from build123d import *

# Parameters (mm, degrees)
SKETCH1_W                        = 45
SKETCH1_H                        = 115
BASE_FLANGE1_DEPTH               = 2
EDGE_FLANGE1_STRIP_W             = 9.9732
EDGE_FLANGE1_STRIP_H             = 2
EDGE_FLANGE1_STRIP_CUT_DEPTH     = 115
EDGE_FLANGE1_DEPTH               = 115
EDGE_FLANGE2_STRIP_W             = 9.9732
EDGE_FLANGE2_STRIP_H             = 2
EDGE_FLANGE2_STRIP_CUT_DEPTH     = 115
EDGE_FLANGE2_DEPTH               = 115
EDGE_FLANGE3_STRIP_W             = 9.9732
EDGE_FLANGE3_STRIP_H             = 2
EDGE_FLANGE3_STRIP_CUT_DEPTH     = 115
EDGE_FLANGE3_DEPTH               = 115
EDGE_FLANGE4_STRIP_W             = 9.9732
EDGE_FLANGE4_STRIP_H             = 2
EDGE_FLANGE4_STRIP_CUT_DEPTH     = 115
EDGE_FLANGE4_DEPTH               = 115
TAP_DRILL_FOR_M5_TAP1_AT_2_COUNT = 2
TAP_DRILL_FOR_M5_TAP1_AT_2_PITCH = 20
TAP_DRILL_FOR_M5_TAP1_AT_3_COUNT = 2
TAP_DRILL_FOR_M5_TAP1_AT_3_PITCH = 69.48
TAP_DRILL_FOR_M5_TAP1_AT_4_COUNT = 2
TAP_DRILL_FOR_M5_TAP1_AT_4_PITCH = 89.48
TAP_DRILL_FOR_M5_TAP1_AT_5_COUNT = 2
TAP_DRILL_FOR_M5_TAP1_AT_5_PITCH = 114.373614001
TAP_DRILL_FOR_M5_TAP1_AT_6_COUNT = 2
TAP_DRILL_FOR_M5_TAP1_AT_6_PITCH = 99.509414527
TAP_DRILL_FOR_M5_TAP1_AT_7_COUNT = 2
TAP_DRILL_FOR_M5_TAP1_AT_7_PITCH = 73.990899302
TAP_DRILL_FOR_M5_TAP1_AT_8_COUNT = 2
TAP_DRILL_FOR_M5_TAP1_AT_8_PITCH = 71.2366


# Sheet-metal steps are written as plain solids
with BuildPart() as part:
    # Sketch1 → Base-Flange1 (new body)
    with BuildSketch(Plane.XY):
        Rectangle(SKETCH1_W, SKETCH1_H)
    extrude(amount=-BASE_FLANGE1_DEPTH)

    # Edge-Flange1 strip (across the edge) → Edge-Flange1 strip cut (cut)
    with BuildSketch(Plane(origin=(23, 57.5, -2), x_dir=(-1, 0, 0), z_dir=(0, -1, 0))):
        with Locations((-4.25, -1)):
            Rectangle(EDGE_FLANGE1_STRIP_W, EDGE_FLANGE1_STRIP_H)
    extrude(amount=EDGE_FLANGE1_STRIP_CUT_DEPTH, mode=Mode.SUBTRACT)

    # Edge-Flange1 section (across the edge) → Edge-Flange1 (add)
    with BuildSketch(Plane(origin=(23, 57.5, -2), x_dir=(-1, 0, 0), z_dir=(0, -1, 0))):
        with BuildLine():
            Line((-2, 0.7366), (-2, 43))
            Line((-2, 43), (0, 43))
            Line((0, 43), (0, 0.7366))
            ThreePointArc((0, 0.7366), (0.215745145, 0.215745145), (0.7366, 0))
            Line((0.7366, 0), (0.7366, -2))
            ThreePointArc((0.7366, -2), (-1.198468417, -1.198468417), (-2, 0.7366))
        make_face()
    extrude(amount=EDGE_FLANGE1_DEPTH)

    # Edge-Flange2 strip (across the edge) → Edge-Flange2 strip cut (cut)
    with BuildSketch(Plane(origin=(25, -57.5, -45.5), x_dir=(0, 0, 1), z_dir=(0, 1, 0))):
        with Locations((-4.25, -1)):
            Rectangle(EDGE_FLANGE2_STRIP_W, EDGE_FLANGE2_STRIP_H)
    extrude(amount=EDGE_FLANGE2_STRIP_CUT_DEPTH, mode=Mode.SUBTRACT)

    # Edge-Flange2 section (across the edge) → Edge-Flange2 (add)
    with BuildSketch(Plane(origin=(25, -57.5, -45.5), x_dir=(0, 0, 1), z_dir=(0, 1, 0))):
        with BuildLine():
            Line((-2, 0.7366), (-2, 20.5))
            Line((-2, 20.5), (0, 20.5))
            Line((0, 20.5), (0, 0.7366))
            ThreePointArc((0, 0.7366), (0.215745145, 0.215745145), (0.7366, 0))
            Line((0.7366, 0), (0.7366, -2))
            ThreePointArc((0.7366, -2), (-1.198468417, -1.198468417), (-2, 0.7366))
        make_face()
    extrude(amount=EDGE_FLANGE2_DEPTH)

    # Edge-Flange3 strip (across the edge) → Edge-Flange3 strip cut (cut)
    with BuildSketch(Plane(origin=(-23, -57.5, -2), x_dir=(1, 0, 0), z_dir=(0, 1, 0))):
        with Locations((-4.25, -1)):
            Rectangle(EDGE_FLANGE3_STRIP_W, EDGE_FLANGE3_STRIP_H)
    extrude(amount=EDGE_FLANGE3_STRIP_CUT_DEPTH, mode=Mode.SUBTRACT)

    # Edge-Flange3 section (across the edge) → Edge-Flange3 (add)
    with BuildSketch(Plane(origin=(-23, -57.5, -2), x_dir=(1, 0, 0), z_dir=(0, 1, 0))):
        with BuildLine():
            Line((-2, 0.7366), (-2, 43))
            Line((-2, 43), (0, 43))
            Line((0, 43), (0, 0.7366))
            ThreePointArc((0, 0.7366), (0.215745145, 0.215745145), (0.7366, 0))
            Line((0.7366, 0), (0.7366, -2))
            ThreePointArc((0.7366, -2), (-1.198468417, -1.198468417), (-2, 0.7366))
        make_face()
    extrude(amount=EDGE_FLANGE3_DEPTH)

    # Edge-Flange4 strip (across the edge) → Edge-Flange4 strip cut (cut)
    with BuildSketch(Plane(origin=(-25, 57.5, -45.5), x_dir=(0, 0, 1), z_dir=(0, -1, 0))):
        with Locations((-4.25, -1)):
            Rectangle(EDGE_FLANGE4_STRIP_W, EDGE_FLANGE4_STRIP_H)
    extrude(amount=EDGE_FLANGE4_STRIP_CUT_DEPTH, mode=Mode.SUBTRACT)

    # Edge-Flange4 section (across the edge) → Edge-Flange4 (add)
    with BuildSketch(Plane(origin=(-25, 57.5, -45.5), x_dir=(0, 0, 1), z_dir=(0, -1, 0))):
        with BuildLine():
            Line((-2, 0.7366), (-2, 20.5))
            Line((-2, 20.5), (0, 20.5))
            Line((0, 20.5), (0, 0.7366))
            ThreePointArc((0, 0.7366), (0.215745145, 0.215745145), (0.7366, 0))
            Line((0.7366, 0), (0.7366, -2))
            ThreePointArc((0.7366, -2), (-1.198468417, -1.198468417), (-2, 0.7366))
        make_face()
    extrude(amount=EDGE_FLANGE4_DEPTH)

    # Sketch21 → Tap Drill for M5 Tap1 (revolve, cut)
    with BuildSketch(Plane(origin=(-35.6183, 44.74, -45.5), x_dir=(0, -1, 0), z_dir=(1, 0, 0))):
        Polygon((0, 0), (0, 2), (2.1, 2), (2.1, 0.025), (2.125, 0), align=None)
    tap_drill_for_m5_tap1 = revolve(axis=Axis((-35.6183, 44.74, -39.15), (0, 0, -1)), mode=Mode.SUBTRACT)

    # Tap Drill for M5 Tap1 at 2: Tap Drill for M5 Tap1 ×2
    with Locations(*[(0, -i * TAP_DRILL_FOR_M5_TAP1_AT_2_PITCH, 0) for i in range(1, TAP_DRILL_FOR_M5_TAP1_AT_2_COUNT)]):
        add(tap_drill_for_m5_tap1, mode=Mode.SUBTRACT)

    # Tap Drill for M5 Tap1 at 3: Tap Drill for M5 Tap1 ×2
    with Locations(*[(0, -i * TAP_DRILL_FOR_M5_TAP1_AT_3_PITCH, 0) for i in range(1, TAP_DRILL_FOR_M5_TAP1_AT_3_COUNT)]):
        add(tap_drill_for_m5_tap1, mode=Mode.SUBTRACT)

    # Tap Drill for M5 Tap1 at 4: Tap Drill for M5 Tap1 ×2
    with Locations(*[(0, -i * TAP_DRILL_FOR_M5_TAP1_AT_4_PITCH, 0) for i in range(1, TAP_DRILL_FOR_M5_TAP1_AT_4_COUNT)]):
        add(tap_drill_for_m5_tap1, mode=Mode.SUBTRACT)

    # Tap Drill for M5 Tap1 at 5: Tap Drill for M5 Tap1 ×2
    with Locations(*[Vector(0.622841208809067, -0.7823482783321378, 0) * (i * TAP_DRILL_FOR_M5_TAP1_AT_5_PITCH) for i in range(1, TAP_DRILL_FOR_M5_TAP1_AT_5_COUNT)]):
        add(tap_drill_for_m5_tap1, mode=Mode.SUBTRACT)

    # Tap Drill for M5 Tap1 at 6: Tap Drill for M5 Tap1 ×2
    with Locations(*[Vector(0.7158779934382821, -0.6982253923417416, 0) * (i * TAP_DRILL_FOR_M5_TAP1_AT_6_PITCH) for i in range(1, TAP_DRILL_FOR_M5_TAP1_AT_6_COUNT)]):
        add(tap_drill_for_m5_tap1, mode=Mode.SUBTRACT)

    # Tap Drill for M5 Tap1 at 7: Tap Drill for M5 Tap1 ×2
    with Locations(*[Vector(0.9627751611583101, -0.27030351284544973, 0) * (i * TAP_DRILL_FOR_M5_TAP1_AT_7_PITCH) for i in range(1, TAP_DRILL_FOR_M5_TAP1_AT_7_COUNT)]):
        add(tap_drill_for_m5_tap1, mode=Mode.SUBTRACT)

    # Tap Drill for M5 Tap1 at 8: Tap Drill for M5 Tap1 ×2
    with Locations(*[(i * TAP_DRILL_FOR_M5_TAP1_AT_8_PITCH, 0, 0) for i in range(1, TAP_DRILL_FOR_M5_TAP1_AT_8_COUNT)]):
        add(tap_drill_for_m5_tap1, mode=Mode.SUBTRACT)


solid = part.part
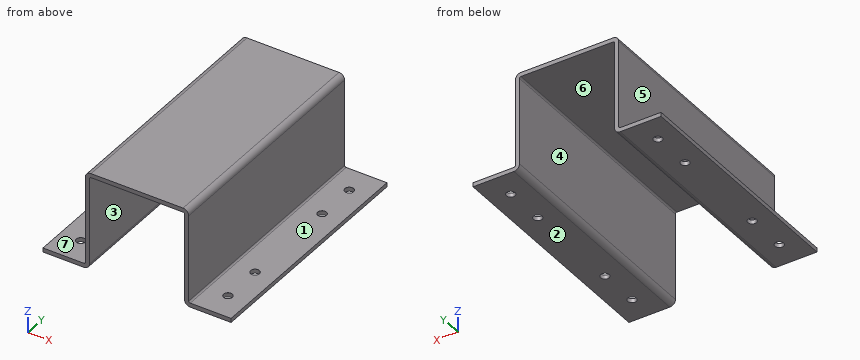
Source: CAD feature listing. Evaluate the final solid. Frame: model axes, mm. Face numbers are marked on the shaded views. A direction names the side the tool comes from. Coordinates: 2 decimals unless noted, no trailing zeros. Order: outer loops, then holes, each group sorted by start corner. A loop starts at its lowest first (then second) coordinate and runs counter-clockwise, first axis right, second up.
Item 1: First-contact query: P1, Ø10, axis at x = 37.5, y = 1, coming from the +Z side; P2, Ø10, axis at y = 42.5, z = -33.5, coming from the +X side; P3, Ø8, axis at y = 39, z = -17.5, coming from the -X side. Flat tips, straight axial feed; report the tip coordinate or a pass-through.
Output values:
P1: stops at z = -45.5
P2: stops at x = 25
P3: stops at x = -25
Item 2: Cut plane C-C (y = -20.5). Return loops of the section in (x, z).
Output values:
outline: (-45.5, -47.5) - (-25.74, -47.5) arc R2.74 ccw to (-23, -44.76) - (-23, -2.74) arc R0.74 cw to (-22.26, -2) - (22.26, -2) arc R0.74 cw to (23, -2.74) - (23, -44.76) arc R2.74 ccw to (25.74, -47.5) - (45.5, -47.5) - (45.5, -45.5) - (25.74, -45.5) arc R0.74 cw to (25, -44.76) - (25, -2.74) arc R2.74 ccw to (22.26, 0) - (-22.26, 0) arc R2.74 ccw to (-25, -2.74) - (-25, -44.76) arc R0.74 cw to (-25.74, -45.5) - (-45.5, -45.5) - close
Item 3: Cut plane B-B (z = -13). Return loops of the section in (x, y), plus the area to 3 significant figures.
Output values:
outline: (-25, -57.5) - (-23, -57.5) - (-23, 57.5) - (-25, 57.5) - close; (23, -57.5) - (25, -57.5) - (25, 57.5) - (23, 57.5) - close
area: 460 mm2
Item 4: Pull-direction query (X, two-part tool) for the marked faces 4, 5, 6 and 7; classes: pulls with the +X half, pulls with the -X half, needs draft (parallel to the pull), parting line crosses it, or undercut.
Output values:
face 4: undercut
face 5: pulls with the -X half
face 6: undercut
face 7: needs draft
Item 5: Cut plane D-D (x = 27). Return loops of the section in (y, z).
Output values:
outline: (-57.5, -47.5) - (57.5, -47.5) - (57.5, -45.5) - (-57.5, -45.5) - close
Item 6: Cut plane A-A (y = 24.74). Count the separate pieces of the cut face and the enclosed holes in it, plus the area to 3 significant figures.
Output values:
separate pieces: 3
enclosed holes: 0
area: 341 mm2
Item 7: Set-up query: the marked faces 1, 2 and 3. Return all of +Z, -Z, +X, -X, +Y, -Y with unobstructed straight access to the full face (end or side cutting, diameter ignored); none if empty.
Output values:
face 1: +Z, +X, +Y, -Y
face 2: -Z, +X, -X, +Y, -Y
face 3: -Z, +Y, -Y
Item 8: Material intervals for line 1 (X direction, y = 48, z = -36.5); line 2 (X direction, y = -24, z = -46); line 3 (Z direction, x = -20, y = -38), sorted ascending.
Output values:
line 1: x = -25 to -23, 23 to 25
line 2: x = -45.5 to -37.58, -33.65 to -23.3, 23.3 to 33.65, 37.58 to 45.5
line 3: z = -2 to 0
